Could you check a few things on this drawing? It's one solid part, dimensions in mm from its lowest x, y, z. A direction names the side the tool comes from. Give positions to 0.01 mm unless a question says otherwise; leave off trailing zeros. Write each loop counter-clockwise with the first axis right and the second up, starting at its lowest first coordinate (ties: lowest second). Pieces come first, ordered by that corner, then holes. Notation, with made-up numbers: (-7, 42.25) -> (42, 42.25) arc R26 cw to (42, 78.25) -> close; hole circle Ø11 at (88, 18.5). An arc over 180 degrees is marked (long way). Answer as CSV lines item,"result". Start each with the question number.
1. If we section it at C-C on z = 21.5: Write out the boundary of the cut face in (x, y).
2. If we section it at D-D on x = 37.5: Write out the boundary of the cut face in (y, z), plus the area to 3 significant figures.
3. If we section it at A-A on x = 16: Write out the boundary of the cut face in (y, z).
4. If we section it at B-B on y = 25: Write out the boundary of the cut face in (x, z), plus the area to 3 significant figures.
5. I'm going to push flat-ended pins straight in: P1, Ø6, axis at x = 30.5, y = 3, coming from the -Z side; P2, Ø3.5, axis at y = 6, z = 22, coming from the -X side; P3, Ø15.5, axis at x = 33.5, z = 19.5, coming from the +Y side; P4, Ø13, axis at x = 35, y = 6.5, coming from the +Z side. Where does each tip first touch, or does it pass through?
6. On a 3-axis mill with a long thin cutter (end or side, diameter ignored), from which of +Z, -Z, +X, -X, +Y, -Y can I reach the whole of each face in a straight line? I mean the marked faces 1, 2, 3 and 4. Say none if no direction works.
7. I need wall thicknesses on line 1 (Y direction, x = 26, z = 7.5); line 2 (Y direction, x = 44, z = 27.5); line 3 (X direction, y = 14, z = 20.5). Which ranges of each line are inside material? Lowest first, please. Write a range as [from, to].
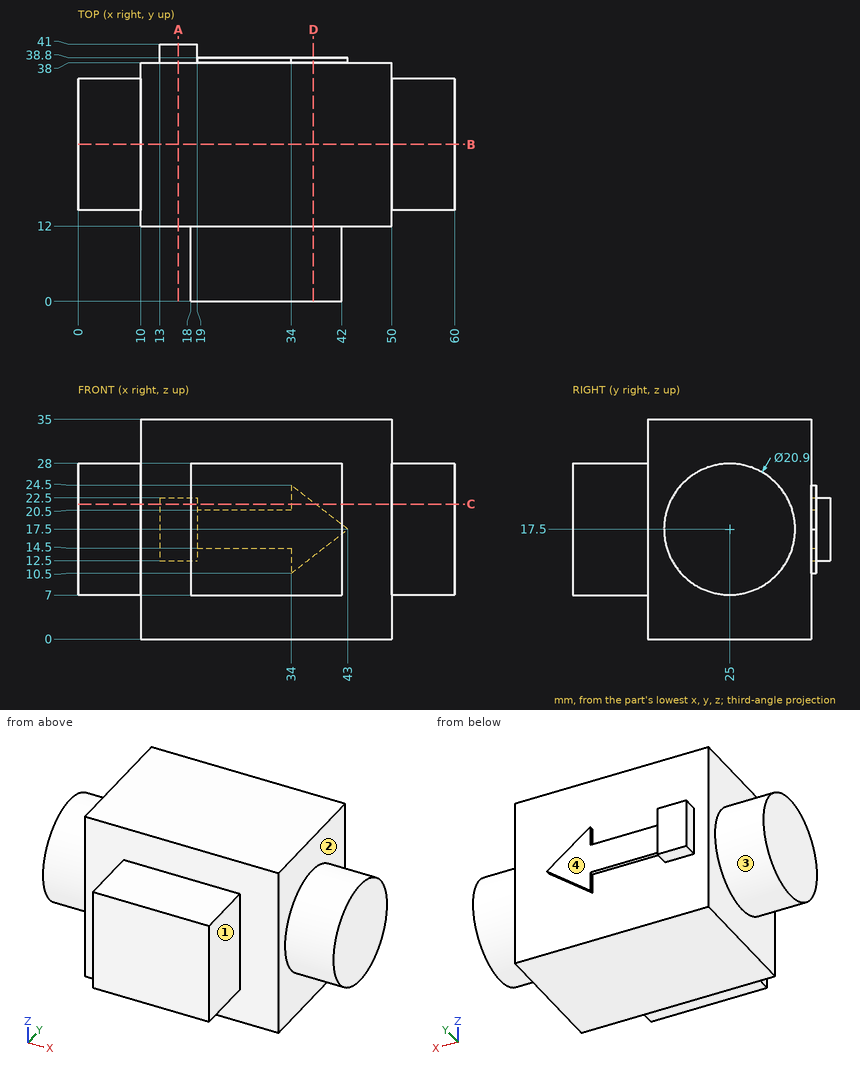
Computed values:
1,outline,"(0, 15.35) -> (10, 15.35) -> (10, 12) -> (18, 12) -> (18, 0) -> (42, 0) -> (42, 12) -> (50, 12) -> (50, 15.35) -> (60, 15.35) -> (60, 34.65) -> (50, 34.65) -> (50, 38) -> (37.86, 38) -> (37.86, 38.8) -> (34, 38.8) -> (34, 38) -> (19, 38) -> (19, 41) -> (13, 41) -> (13, 38) -> (10, 38) -> (10, 34.65) -> (0, 34.65) -> close"
2,outline,"(0, 7) -> (12, 7) -> (12, 0) -> (38, 0) -> (38, 13.22) -> (38.8, 13.22) -> (38.8, 21.78) -> (38, 21.78) -> (38, 35) -> (12, 35) -> (12, 28) -> (0, 28) -> close"
2,area,"1,170 mm2"
3,outline,"(12, 0) -> (38, 0) -> (38, 12.5) -> (41, 12.5) -> (41, 22.5) -> (38, 22.5) -> (38, 35) -> (12, 35) -> close"
4,outline,"(0, 7.05) -> (10, 7.05) -> (10, 0) -> (50, 0) -> (50, 7.05) -> (60, 7.05) -> (60, 27.95) -> (50, 27.95) -> (50, 35) -> (10, 35) -> (10, 27.95) -> (0, 27.95) -> close"
4,area,"1,820 mm2"
5,P1,"stops at z = 7"
5,P2,"stops at x = 18"
5,P3,"stops at y = 38.8"
5,P4,"stops at z = 35"
6,face 1,"+Z, -Z, +X, -Y"
6,face 2,"+X"
6,face 3,"-X"
6,face 4,"+Z, -Z, +X, +Y"
7,line 1,"y = [0, 38]"
7,line 2,"y = [12, 38]"
7,line 3,"x = [10, 50]"
